```python
from build123d import *

# Parameters (mm, degrees)
SKETCH1_R           = 2.75
BOSS_EXTRUDE1_DEPTH = 2


with BuildPart() as part:
    # Sketch1 → Boss-Extrude1 (new body)
    with BuildSketch(Plane.XY):
        Polygon((0, 98), (0, 2), (2, 0), (18, 0), (100, 82), (100, 98), (98, 100), (2, 100), align=None)
        with Locations((91, 91)):
            Circle(SKETCH1_R, mode=Mode.SUBTRACT)
        with Locations((28, 91)):
            Circle(SKETCH1_R, mode=Mode.SUBTRACT)
        with Locations((9, 9)):
            Circle(SKETCH1_R, mode=Mode.SUBTRACT)
        with Locations((9, 72)):
            Circle(SKETCH1_R, mode=Mode.SUBTRACT)
    extrude(amount=-BOSS_EXTRUDE1_DEPTH)


solid = part.part
```
Source: CAD feature listing. Evaluate the final solid. Frame: model axes, mm. Round coordinates to 2 decimals unless told otherwise and drop trailing zeros. Loops run counter-clockwise (first coordinate to the right, second up) from the corner with the lowest first, then second, coordinate; pieces in that order, holes last.
(1) Pull-direction query (Y, two-part tool) for faces 1 (the flat face through (38, 62, 0)), 2 (the flat face through (58, 40, -1)), 3 (the cylindrical face through (8.642, 11.727, -0.986)), 4 (the cylindrical face through (25.818, 89.327, -0.986)); classes: +Y half, -Y half, draft (parallel to the pull), parting line (faces both ways), or undercut.
From the geometry:
face 1: draft
face 2: -Y half
face 3: undercut
face 4: undercut
(2) Material intervals for probe 1 along Y at (x, z) = (9, -0.9); probe 2 along Y at (x, z) = (10, -1.5); probe 3 along Y at (x, z) = (20, -1.85), sorted ascending.
From the geometry:
probe 1: y = 0 to 6.25, 11.75 to 69.25, 74.75 to 100
probe 2: y = 0 to 6.44, 11.56 to 69.44, 74.56 to 100
probe 3: y = 2 to 100
(3) Section query B-B (y = 72). Output: boundary loops of the cut face in (x, z), and give its area (3 significant figures).
From the geometry:
outline: (0, -2) - (6.25, -2) - (6.25, 0) - (0, 0) - close; (11.75, -2) - (90, -2) - (90, 0) - (11.75, 0) - close
area: 169 mm2
(4) Section query C-C (x = 9). Output: boundary loops of the cut face in (y, z), and give its area (3 significant figures).
From the geometry:
outline: (0, -2) - (6.25, -2) - (6.25, 0) - (0, 0) - close; (11.75, -2) - (69.25, -2) - (69.25, 0) - (11.75, 0) - close; (74.75, -2) - (100, -2) - (100, 0) - (74.75, 0) - close
area: 178 mm2
(5) Section query A-A (x = 28). Output: boundary loops of the cut face in (y, z), and give its area (3 significant figures).
From the geometry:
outline: (10, -2) - (88.25, -2) - (88.25, 0) - (10, 0) - close; (93.75, -2) - (100, -2) - (100, 0) - (93.75, 0) - close
area: 169 mm2
(6) Section query D-D (y = 91). Output: boundary loops of the cut face in (x, z), and give its area (3 significant figures).
From the geometry:
outline: (0, -2) - (25.25, -2) - (25.25, 0) - (0, 0) - close; (30.75, -2) - (88.25, -2) - (88.25, 0) - (30.75, 0) - close; (93.75, -2) - (100, -2) - (100, 0) - (93.75, 0) - close
area: 178 mm2
(7) Contact query for a flat-ended pin moving along its axis: pin 1 Ø1 at (x, z) = (79, -1) entering from -Y. Output: stop coordinate, or through.
From the geometry:
pin 1: stops at y = 60.5
